Build history of the part. All positions in model axes, mm. A direction names the side the tool comes from. Round coordinates to 2 decimals unless told otherwise and drop trailing zeros. Write each loop counter-clockwise with the first axis right and the second up, starting at its lowest first coordinate (ties: lowest second). Pieces come first, ordered by that corner, then holes. Notation, with made-up numbers: (0.5, 61) - (43.5, 61) arc R30 cw to (43.5, 85) - close; hole circle Ø6 at (-24, 85.5). An arc over 180 degrees is marked (long way). Answer as a JSON object with one key per item and string values. Group by question number.
Item 1: Probe line 1 (X direction, y = -1.75, z = 43.5); line 2 (Z direction, x = 63, y = -0.5); line 3 (Z direction, x = 94.5, y = -1.7). List the from-to ranges inside material, lowest first. Write a range as from..to.
Item 2: Two-plate mould, pull along X, no slides. Class faces 3 (the cylindrical face through (74.51, -1.52, 95.72)), 4 (the flat face through (50, -1, 25.825)), 5 (the flat face through (72, -3, 51)), 6 (the flat face through (100, -1, 42)): +X half, -X half, draft (parallel to the pull), parting line (faces both ways), or undercut.
Item 3: Slice it at C-C, the plane z = 86.5. List the corners of the cut face in (x, y), then the cut area to 3 significant figures.
Item 4: Which spindle directions (+Z, -Z, +X, -X, +Y, -Y) get a long thin tool onto all of the face, cutting with end or side? Do faces 1 (the flat face through (30, -1, 55)), 2 (the flat face through (72, 0, 51)). Say none if no direction does.
Item 5: Slice it at A-A, the plane z = 59.5. List the corners of the cut face in (x, y).
Item 6: Slice it at D-D, the plane x = 40.5. List the corners of the cut face in (y, z).
Item 7: Flat gauge pin, fed straight in: pin 1 (0.9 mm diameter, centred on x = 42, y = -2, fed in from +Z). Where does the tip first touch, or does it go through?
from build123d import *

# Parameters (mm, degrees)
F1_DEPTH = 3
F2_R     = 14.99999


# Not quite as in the source:
# - a fillet or chamfer is up to 0.001 mm smaller than in the source, because OpenCascade refuses the exact size


with BuildPart() as f1:
    # F0 (on Front) → F1 (new body)
    with BuildSketch(Plane.XZ):
        Polygon((0, 25.8250685402), (0, 0), (100, 0), (100, 25.8250685402), (100, 100), (70, 100), (70, 25.8250685402), (30, 25.8250685402), (30, 100), (0, 100), align=None)
    extrude(amount=F1_DEPTH)

    # F2 (radius 15 in the source; OpenCascade refuses exactly that, so slightly less here)
    f2_edges = [f1.edges().sort_by_distance(p)[0] for p in [
        (100, -1.5, 100),
        (70, -1.5, 100),
        (30, -1.5, 100),
        (0, -1.5, 100),
    ]]
    fillet(f2_edges, radius=F2_R)


solid = f1.part
Geometry says:
{
 "1": {"line 1": "x = 0..30, 70..100", "line 2": "z = 0..25.83", "line 3": "z = 0..96.61"},
 "2": {"face 3": "undercut", "face 4": "undercut", "face 5": "draft", "face 6": "+X half"},
 "3": {"outline": "(0.08, -3) - (29.92, -3) - (29.92, 0) - (0.08, 0) - close; (70.08, -3) - (99.92, -3) - (99.92, 0) - (70.08, 0) - close", "area": "179 mm^2"},
 "4": {"face 1": "+Z, +Y, -Y", "face 2": "+Z, -Z, +X, -X, +Y"},
 "5": {"outline": "(0, -3) - (30, -3) - (30, 0) - (0, 0) - close; (70, -3) - (100, -3) - (100, 0) - (70, 0) - close"},
 "6": {"outline": "(-3, 0) - (0, 0) - (0, 25.83) - (-3, 25.83) - close"},
 "7": {"pin 1": "stops at z = 25.83"}
}
